from build123d import *

# Parameters (mm, degrees)
F0_R         = 7.5
F0_R_2       = 2.5
F1_DEPTH     = 200
F2_R         = 1.5
F3_DEPTH     = 25
F4_W         = 255.6320726871
F4_H         = 34.7503256053
F5_DEPTH     = 25
F6_W         = 10
F6_H         = 5
F6_H_2       = 4.8793365061
F7_DEPTH     = 4
F8_R         = 1.75
F9_DEPTH     = 7.501
F11_DEPTH    = 20
F12_T2_ANGLE = 359.64
F12_T4_ANGLE = 359.64


# Not quite as in the source:
# - a fillet or chamfer that OpenCascade refuses, or shapes differently, is made with other operations: its cross-section is extruded or revolved along the edge and cut away or added


with BuildPart() as f1:
    # F0 (on Front) → F1 (new body)
    with BuildSketch(Plane.XZ):
        Circle(F0_R)
        Circle(F0_R_2, mode=Mode.SUBTRACT)
    extrude(amount=-F1_DEPTH)

    # F2 (on face) → F3 (cut)
    with BuildSketch(Plane.XZ):
        with Locations((5, 0)):
            Circle(F2_R)
        with Locations((-5, 0)):
            Circle(F2_R)
    extrude(amount=-F3_DEPTH, mode=Mode.SUBTRACT)

    # F4 (on Right) → F5 (cut)
    with BuildSketch(Plane.YZ):
        with Locations((127.8160363436, -0.9753750637)):
            Rectangle(F4_W, F4_H)
    extrude(amount=F5_DEPTH, mode=Mode.SUBTRACT)

    # F6 (on face) → F7 (join)
    with BuildSketch(Plane.YZ):
        with BuildLine():
            ThreePointArc((10, 7.5), (5, 12.5), (0, 7.5))
            Line((0, 7.5), (10, 7.5))
        make_face()
        with Locations((5, 5)):
            Rectangle(F6_W, F6_H)
        with BuildLine():
            Line((190, 7.5), (200, 7.5))
            ThreePointArc((200, 7.5), (195, 12.5), (190, 7.5))
        make_face()
        with Locations((195, 5)):
            Rectangle(F6_W, F6_H)
        with BuildLine():
            ThreePointArc((190, -7.5), (195, -12.5), (200, -7.5))
            Line((200, -7.5), (190, -7.5))
        make_face()
        with Locations((195, -5.0603317469)):
            Rectangle(F6_W, F6_H_2)
        with BuildLine():
            Line((10, -7.5), (0, -7.5))
            ThreePointArc((0, -7.5), (5, -12.5), (10, -7.5))
        make_face()
        with Locations((5, -5.0603317469)):
            Rectangle(F6_W, F6_H_2)
    extrude(amount=-F7_DEPTH)

    # F8 (on face) → F9 (cut, through all)
    with BuildSketch(Plane.YZ):
        with Locations((5, 10)):
            Circle(F8_R)
        with Locations((5, -10)):
            Circle(F8_R)
        with Locations((195, 10)):
            Circle(F8_R)
        with Locations((195, -10)):
            Circle(F8_R)
    extrude(amount=-F9_DEPTH, mode=Mode.SUBTRACT)

    # F10 (on face) → F11 (join)
    with BuildSketch(Plane(origin=(0, 200, 0), x_dir=(-1, 0, 0), z_dir=(0, 1, 0))):
        with BuildLine():
            Line((0, 2.5), (0, 2))
            ThreePointArc((0, 2), (2, 0), (0, -2))
            Line((0, -2), (0, -2.5))
            ThreePointArc((0, -2.5), (2.5, 0), (0, 2.5))
        make_face()
    extrude(amount=-F11_DEPTH)

    # F12: fillet of radius 2 on 2 edges, made by hand

    # F12_s1 → F12_t2 (revolve, cut)
    with BuildSketch(Plane(origin=(0, 0, 0), x_dir=(0, 1, 0), z_dir=(0.0031415875, 0, -0.9999950652))):
        with BuildLine():
            ThreePointArc((198, 2), (199.4142135624, 2.5857864376), (200, 4))
            Line((200, 4), (200, 2))
            Line((200, 2), (198, 2))
        make_face()
    revolve(axis=Axis((0, 200, 0), (0, -1, 0)), revolution_arc=F12_T2_ANGLE, mode=Mode.SUBTRACT)

    # F12_s3 → F12_t4 (revolve, cut)
    with BuildSketch(Plane(origin=(0, 0, 0), x_dir=(0, 1, 0), z_dir=(0.0031415875, 0, -0.9999950652))):
        with BuildLine():
            ThreePointArc((180, 2.5), (180.6157688743, 2.1291713066), (181.3228756555, 2))
            Line((181.3228756555, 2), (180, 2))
            Line((180, 2), (180, 2.5))
        make_face()
    revolve(axis=Axis((0, 180, 0), (0, -1, 0)), revolution_arc=F12_T4_ANGLE, mode=Mode.SUBTRACT)


solid = f1.part
The model under review builds one solid part; all positions refer to its coordinate system, in mm. A direction names the side the tool comes from. Coordinates: 2 decimals unless noted, no trailing zeros. Write each loop counter-clockwise with the first axis right and the second up, starting at its lowest first coordinate (ties: lowest second). Pieces come first, ordered by that corner, then holes. Notation, with made-up numbers: M 46,63 L 99,63 A20 ccw 99,83 Z; hole C 26,65 d9. An arc over 180 degrees is marked long. Put each result on its own line as item: value.
1) For faces 1 (the flat face through (0, 101, -5)), 2 (the flat face through (-4, 5, 8)), 3 (the flat face through (-4, 5, -8)), list the 3-axis set-ups (+Z, -Z, +X, -X, +Y, -Y) from which the entire face can be reached by the end or side of a thin tool; tool diameter is ignored.
Computed:
face 1: +Z, -Z, +X, +Y, -Y
face 2: +Z, -X, +Y, -Y
face 3: -Z, -X, +Y, -Y
2) Add section C-C on y = 177.5. Give the boundary of the cut face in (x, z), then the cut area to 3 significant figures.
Computed:
outline: M 0,-7.5 L 0,-2.5 A2.5 cw 0,2.5 L 0,7.5 A7.5 ccw Z
area: 78.5 mm2
3) Add section D-D on x = -5.25. Give the boundary of the cut face in (y, z).
Computed:
outline: M 0,-5.36 L 200,-5.36 L 200,5.36 L 0,5.36 L 0,1.48 L 25,1.48 L 25,-1.48 L 0,-1.48 Z
4) Draft analysis for pull direction Z (two halves, no side actions). For faces 4 (the cylindrical face through (-7.5, 98.6, 0.16)), 5 (the flat face through (-4, 195, -8)), 6 (the cylindrical face through (-1.972, 196.669, -9.474)), state which applies: released by +Z, released by -Z, zero draft, split by the parting line, or undercut.
Computed:
face 4: split by the parting line
face 5: zero draft
face 6: undercut
5) Wall thickness on probe 1 along Y at (x, z) = (-3.25, 10.5); probe 2 along Z at (x, y) = (-2.2, 5); probe 3 along Z at (x, y) = (-5, 9.5): over which ranges is each line inside the solid? List them lowest first. Write a range as [from, to].
Computed:
probe 1: y = [1, 3.32], [6.68, 9], [191, 193.32], [196.68, 199]
probe 2: z = [-12.5, -11.75], [-8.25, -1.19], [1.19, 8.25], [11.75, 12.5]
probe 3: z = [-5.59, -1.5], [1.5, 5.59]
6) Add section B-B on z = -10. Give the boundary of the cut face in (x, y).
Computed:
outline: M -4,0.67 L 0,0.67 L 0,3.25 L -4,3.25 Z; M -4,6.75 L 0,6.75 L 0,9.33 L -4,9.33 Z; M -4,190.67 L 0,190.67 L 0,193.25 L -4,193.25 Z; M -4,196.75 L 0,196.75 L 0,199.33 L -4,199.33 Z
7) Clearance check with flat-ended pins moving along their axes: pin 1 Ø5.5 at (y, z) = (5, -10) entering from +X; pin 2 Ø1 at (x, y) = (-3, 69) entering from -Z; pin 3 Ø8 at (y, z) = (130, 8) entering from -X; pin 4 Ø1 at (x, y) = (-4.5, 69) entering from +Z. State where each tip first meets the part, or that it passes through.
Computed:
pin 1: stops at x = 0
pin 2: stops at z = -7.07
pin 3: stops at x = -6.34
pin 4: stops at z = 6.34
8) Add section A-A on y = 5. Give the boundary of the cut face in (x, z), then the cut area to 3 significant figures.
Computed:
outline: M -4,-12.5 L 0,-12.5 L 0,-11.75 L -4,-11.75 Z; M -4,-8.25 L 0,-8.25 L 0,-2.5 A2.5 cw 0,2.5 L 0,8.25 L -4,8.25 L -4,6.34 A7.5 ccw -4,-6.34 Z; M -4,11.75 L 0,11.75 L 0,12.5 L -4,12.5 Z; hole C -5,0 d3
area: 86.5 mm2
